```python
from build123d import *

# Parameters (mm, degrees)
SALIENTE_EXTRUIR1_DEPTH = 25
CORTAR_EXTRUIR1_DEPTH   = 25
CROQUIS5_W              = 25
CROQUIS5_H              = 25
SALIENTE_EXTRUIR2_DEPTH = 35
VACIADO14_START         = 2
VACIADO14_DEPTH         = 18
CROQUIS14_W             = 15
CROQUIS14_H             = 15
CORTAR_EXTRUIR3_DEPTH   = 37


# Read off the part's stored shape, not the designer's step: Vaciado14
with BuildPart() as part:
    # Croquis1 → Saliente-Extruir1 (new body)
    with BuildSketch(Plane.XY):
        with BuildLine():
            Line((0, 0), (30, 0))
            ThreePointArc((30, 0), (55.704345855, 31.740373797), (70, 70))
            ThreePointArc((70, 70), (49.790199458, 101.721443851), (12.5, 96.809513237))
            Line((12.5, 96.809513237), (12.5, 70))
            Line((12.5, 70), (0, 70))
            Line((0, 70), (-12.5, 70))
            Line((-12.5, 70), (-12.5, 96.809513237))
            ThreePointArc((-12.5, 96.809513237), (-49.790199458, 101.721443851), (-70, 70))
            ThreePointArc((-70, 70), (-55.704345855, 31.740373797), (-30, 0))
            Line((-30, 0), (0, 0))
        make_face()
    extrude(amount=SALIENTE_EXTRUIR1_DEPTH)

    # Croquis2 → Cortar-Extruir1 (cut)
    with BuildSketch(Plane.XY):
        with BuildLine():
            ThreePointArc((25, 50), (12.5, 62.5), (0, 50))
            ThreePointArc((0, 50), (-12.5, 62.5), (-25, 50))
            ThreePointArc((-25, 50), (-15.02993221, 32.891723159), (0, 20))
            ThreePointArc((0, 20), (15.02993221, 32.891723159), (25, 50))
        make_face()
    extrude(amount=CORTAR_EXTRUIR1_DEPTH, mode=Mode.SUBTRACT)

    # Croquis5 → Saliente-Extruir2 (add)
    with BuildSketch(Plane(origin=(0, 70, 0), x_dir=(1, 0, 0), z_dir=(0, 1, 0))):
        with Locations((0, -12.5)):
            Rectangle(CROQUIS5_W, CROQUIS5_H)
    extrude(amount=SALIENTE_EXTRUIR2_DEPTH)

    # Vaciado14 outline → Vaciado14 (cut)
    with BuildSketch(Plane.XY.offset(VACIADO14_START)):
        with BuildLine():
            Line((-28.84831613, 3), (25.844637923, 3))
            ThreePointArc((25.844637923, 3), (52.641551282, 36.515307349), (66.170757203, 77.237671959))
            ThreePointArc((66.170757203, 77.237671959), (41.679167851, 101.2951868), (9.5, 89.332614929))
            Line((9.5, 89.332614929), (9.5, 102))
            Line((9.5, 102), (-9.5, 102))
            Line((-9.5, 102), (-9.5, 89.332614929))
            ThreePointArc((-9.5, 89.332614929), (-45.060390177, 100.377434873), (-66.998683941, 70.290217258))
            ThreePointArc((-66.998683941, 70.290217258), (-53.306904817, 33.592972957), (-28.84831613, 3))
        make_face()
        with BuildLine():
            ThreePointArc((0, 59.16515139), (17.591066798, 64.640049141), (27.989581723, 49.43179402))
            ThreePointArc((27.989581723, 49.43179402), (16.926348915, 30.486291666), (0, 16.528287079))
            ThreePointArc((0, 16.528287079), (-16.926348915, 30.486291666), (-27.989581723, 49.43179402))
            ThreePointArc((-27.989581723, 49.43179402), (-17.591066798, 64.640049141), (0, 59.16515139))
        make_face(mode=Mode.SUBTRACT)
    extrude(amount=VACIADO14_DEPTH, mode=Mode.SUBTRACT)

    # Croquis14 → Cortar-Extruir3 (cut)
    with BuildSketch(Plane(origin=(0, 120, 0), x_dir=(1, 0, 0), z_dir=(0, 1, 0))):
        with Locations((0, -12.5)):
            Rectangle(CROQUIS14_W, CROQUIS14_H)
    extrude(amount=-CORTAR_EXTRUIR3_DEPTH, mode=Mode.SUBTRACT)


solid = part.part
```
For this review, take the finished solid that the model builds, in its own axes (mm). A direction names the side the tool comes from. Coordinates: 2 decimals unless noted, no trailing zeros. Loops run counter-clockwise (first coordinate to the right, second up) from the corner with the lowest first, then second, coordinate; pieces in that order, holes last.
1. For faces 1 (the flat face through (0, 105, 21)), 2 (the flat face through (0, 104, 5)), 3 (the flat face through (-1, 66, 20)), list the 3-axis set-ups (+Z, -Z, +X, -X, +Y, -Y) from which the entire face can be reached by the end or side of a thin tool; tool diameter is ignored.
2. Mouldability with a two-part tool opening along Z and no side actions: class faces 4 (the flat face through (9.5, 96, 11)), 5 (the cylindrical face through (12.775, 62.497, 12.325)) as +Z half, -Z half, draft (parallel to the pull), parting line (faces both ways), or undercut.
3. Insertion check: P1, Ø9, axis at y = 99.5, z = 18, coming from the -X side; P2, Ø2, axis at x = -31.5, z = 3.5, coming from the -Y side; P3, Ø8, axis at y = 64, z = 16.5, coming from the +X side; P4, Ø14.5, axis at x = -0.5, z = 13.5, coming from the +Y side. Each pin has a flat end and moves straight along its axis. Give the tip position at first contact, or say it passes through.
4. Add section C-C, the plane x = 37. Give the boundary of the cut face in (y, z).
5. Add section B-B, the plane z = 7. Give the boundary of the cut face in (x, y), then the cut area to 3 significant figures.
6. For line 1 (Z direction, x = -44, y = 44.5); line 2 (X direction, y = 30, z = 9.25); line 3 (X direction, y = 23, z = 8), list the stretches that pass through material, from the lowest coordinate up.
7. Add section A-A, the plane y = 42. Give the boundary of the cut face in (x, z).
8. Add section D-D, the plane y = 25.5. Give the boundary of the cut face in (x, z), then the cut area to 3 significant figures.
Result:
1. face 1: +Z, -Z, +X, -X, +Y
1. face 2: +Y
1. face 3: none
2. face 4: undercut
2. face 5: draft
3. P1: stops at x = -59.49
3. P2: stops at y = 0.45
3. P3: stops at x = 69.59
3. P4: stops at y = 105
4. outline: (6.74, 0) - (104.94, 0) - (104.94, 25) - (6.74, 25) - close; hole (14.13, 2) - (101.94, 2) - (101.94, 20) - (14.13, 20) - close
5. outline: (-70, 70) arc R126.95 ccw to (-30, 0) - (30, 0) arc R126.95 ccw to (70, 70) arc R35 ccw to (12.5, 96.81) - (12.5, 105) - (7.5, 105) - (7.5, 102) - (9.5, 102) - (9.5, 89.33) arc R32 cw to (66.17, 77.24) arc R121.95 cw to (25.84, 3) - (-28.85, 3) arc R123.95 cw to (-67, 70.29) arc R32 cw to (-9.5, 89.33) - (-9.5, 102) - (-7.5, 102) - (-7.5, 105) - (-12.5, 105) - (-12.5, 96.81) arc R35 ccw to start; (-27.99, 49.43) arc R62.53 ccw to (0, 16.53) arc R62.53 ccw to (27.99, 49.43) arc R15.5 ccw to (0, 59.17) arc R15.5 ccw to start; hole (-25, 50) arc R59.53 ccw to (0, 20) arc R59.53 ccw to (25, 50) arc R12.5 ccw to (0, 50) arc R12.5 ccw to start
5. area: 1,860 mm2
6. line 1: z = 0 to 2, 20 to 25
6. line 2: x = -54.69 to -51.19, -16.51 to -12.46, 12.46 to 16.51, 48.84 to 54.69
6. line 3: x = -50.23 to -46.57, -9.37 to -4.51, 4.51 to 9.37, 44.11 to 50.23
7. outline: (-60.96, 0) - (-21.29, 0) - (-21.29, 25) - (-60.96, 25) - close; (21.29, 0) - (60.96, 0) - (60.96, 25) - (21.29, 25) - close; hole (-57.66, 2) - (-24.7, 2) - (-24.7, 20) - (-57.66, 20) - close; hole (24.7, 2) - (55.44, 2) - (55.44, 20) - (24.7, 20) - close
8. outline: (-51.9, 0) - (-7.68, 0) - (-7.68, 25) - (-51.9, 25) - close; (7.68, 0) - (51.9, 0) - (51.9, 25) - (7.68, 25) - close; hole (-48.3, 2) - (-12.19, 2) - (-12.19, 20) - (-48.3, 20) - close; hole (12.19, 2) - (45.88, 2) - (45.88, 20) - (12.19, 20) - close
8. area: 954 mm2
